Design review of the part built by this model. Coordinates are the model's own, in mm. Give positions to 0.01 mm unless a question says otherwise; leave off trailing zeros. Write each loop counter-clockwise with the first axis right and the second up, starting at its lowest first coordinate (ties: lowest second). Pieces come first, ordered by that corner, then holes. Notation, with made-up numbers: (66.5, 48) - (112.5, 48) arc R17 cw to (112.5, 73) - close; hole circle Ø5 at (32, 56.5). An arc over 180 degrees is marked (long way). Write each question's results on one line, items separated by ' | '. Start each with the question number.
Autodesk Inventor part; units mm, degrees
ref_plane "YZ Plane" through (0, 0, 0) normal (1, 0, 0) x (0, 1, 0)
ref_plane "XZ Plane" through (0, 0, 0) normal (0, 1, 0) x (-1, 0, 0)
ref_plane "XY Plane" through (0, 0, 0) normal (0, 0, 1) x (1, 0, 0)
sketch "Sketch1" plane through (0, 0, 0) normal (0, 1, 0) x (-1, 0, 0)
  circle A0 centre (0, 0) radius 1.5875
  dimension "d0" = 3.175
extrude "Extrusion1" add sketch "Sketch1" along normal blind 254
sketch "Sketch9" plane through (0, 0, 0) normal (1, 0, 0) x (0, 1, 0)
  line L0 (0, -1.5875) -> (0, 1.5875)
  line L1 (254, -1.5875) -> (254, 1.5875)
  line L2 (254, 0) -> (228.6, 0)
  line L3 (0, 0) -> (25.4, 0)
  dimension "d42" = 25.4
  dimension "d43" = 25.4
hole "Hole5" at (0, 25.4, 0) direction (-1, 0, 0) diameter 1.1906 end through all both
hole "Hole6" [suppressed]
sketch "Sketch10" plane through (0, 254, 0) normal (0, 1, 0) x (1, 0, 0)
  circle A0 centre (0, 0) radius 1.5875
hole "Hole7" at (0, 254, 0) direction (0, -1, 0) diameter 1.905 end through all
thread "Thread28"
thread "Thread29"
thread "Thread30"
thread "Thread31"
thread "Thread32"
thread "Thread33"
thread "Thread34"
thread "Thread35"
thread "Thread36"
thread "Thread37"
thread "Thread38"
sketch "Sketch14" plane through (0, 254, 0) normal (0, 1, 0) x (1, 0, 0)
  circle A0 centre (0, 0) radius 1.5875
  circle A1 centre (0, 0) radius 0.9525
extrude "Extrusion3" add sketch "Sketch14" along normal blind 50.8
thread "Thread39"
properties part number "burder_rod_2"
Q1. Insertion check: P1, Ø1, axis at x = 1, y = 112, coming from the +Z side; P2, Ø1.5, axis at y = 25.4, z = 0, coming from the -X side. Each pin has a flat end and moves straight along its axis. Give the tip position at first contact, or say it passes through.
Q2. For line 1 along Y through (x, z) = (-1.15, 0); line 2 along Z through (x, y) = (-0.25, 48); line 3 along Z through (x, y) = (0, 77), list the stretches that pass through material, from the lowest coordinate up. Write a range as [from, to].
Q3. Add section A-A on y = 269.5. State the section outline as (x, z) points (1 decimal).
Result:
1) P1: stops at z = 1.51 | P2: stops at x = -1.59
2) line 1: y = [0, 24.8], [26, 304.8] | line 2: z = [-1.57, -0.92], [0.92, 1.57] | line 3: z = [-1.59, -0.95], [0.95, 1.59]
3) outline: circle Ø3.2 at (0, 0); hole circle Ø1.9 at (0, 0)
